```python
from build123d import *

# Parameters (mm, degrees)
F0_R     = 9.5631
F1_DEPTH = 2.5
F2_R     = 8.9162314004
F2_R_2   = 7.9162314004
F3_DEPTH = 0.5
F4_R     = 4
F5_DEPTH = 3.5
F6_R     = 1.2071067812
F7_R     = 1.975
F8_DEPTH = 2.75
F9_R     = 0.4828427125
F10_R    = 0.4587005769


with BuildPart() as f1:
    # F0 (on Top) → F1 (new body)
    with BuildSketch(Plane.XY):
        Circle(F0_R)
    extrude(amount=F1_DEPTH)

    # F2 (on face) → F3 (cut)
    with BuildSketch(Plane.XY.offset(2.5)):
        Circle(F2_R)
        Circle(F2_R_2, mode=Mode.SUBTRACT)
        Polygon((1.8036346717, 5.9258921407), (-2.7067440096, 5.9258921407), (-2.7067440096, 4.4258921407), (-1.8036346717, 4.4258921407), (-1.8036346717, 3.1822535675), (-5.7792644948, 3.1822535675), (-5.7792644948, -4.3527372181), (-4.1694175287, -4.3527372181), (-4.1694175287, -2.3218090646), (-3.4134816378, -2.3218090646), (-3.4134816378, 0), (-1.8036346717, 0), (-2.0609125495, -6.6612055525), (0, -6.6612055525), (2.0609125495, -6.6612055525), (1.8036346717, 0), (3.4134816378, 0), (3.4134816378, -2.3218090646), (4.1694175287, -2.3218090646), (4.1694175287, -4.3527372181), (5.7792644948, -4.3527372181), (5.7792644948, 3.1822535675), (1.8036346717, 3.1822535675), align=None)
    extrude(amount=-F3_DEPTH, mode=Mode.SUBTRACT)

    # F4 (on face) → F5 (join)
    with BuildSketch(Plane(origin=(0, 0, 0), x_dir=(1, 0, 0), z_dir=(0, 0, -1))):
        Circle(F4_R)
    extrude(amount=F5_DEPTH)

    # F6
    f6_edges = [f1.edges().sort_by_distance(p)[0] for p in [
        (-9.5631, 0, 0),
    ]]
    fillet(f6_edges, radius=F6_R)

    # F7 (on face) → F8 (join)
    with BuildSketch(Plane(origin=(0, 0, -3.5), x_dir=(1, 0, 0), z_dir=(0, 0, -1))):
        Circle(F7_R)
    extrude(amount=F8_DEPTH)

    # F9
    f9_edges = [f1.edges().sort_by_distance(p)[0] for p in [
        (-1.975, 0, -6.25),
    ]]
    fillet(f9_edges, radius=F9_R)

    # F10
    f10_edges = [f1.edges().sort_by_distance(p)[0] for p in [
        (-4, 0, -3.5),
    ]]
    fillet(f10_edges, radius=F10_R)


solid = f1.part
```
Check sheet for the modelled part. Datum: model origin and axes. Units: mm. A direction names the side the tool comes from. Round coordinates to 2 decimals unless told otherwise and drop trailing zeros. Order: outer loops, then holes, each group sorted by start corner. A loop starts at its lowest first (then second) coordinate and runs counter-clockwise, first axis right, second up.
1) Tool access check on faces 4 (the cylindrical face through (9.121, 2.872, 1.845)), 5 (the flat face through (4, 2, 0)), 6 (the flat face through (-1.4, 8, 2)). Record the directions out of +Z, -Z, +X, -X, +Y, -Y that give a thin tool (end or side, any length) a straight path to the whole face; none if there is none.
2) Section check A-A (z = 2.25). Record the boundary of the cut face in (x, y), and give its area (3 significant figures).
3) Section check D-D (z = -0.5). Record the boundary of the cut face in (x, y), and give its area (3 significant figures).
4) Mould release check, pull along X, two halves, no side actions. Record for faces 1 (the cylindrical face through (-1.933, -8.704, 2.254)), 2 (the cylindrical face through (-1.57, 1.2, -4.62)), 3 (the flat face through (3, -2, 2.5)): +X half, -X half, draft (parallel to the pull), parting line (faces both ways), or undercut.
5) Go/stop test with flat-tipped pins: pin 1 Ø3 at (x, z) = (2.5, -1) entering from +Y; pin 2 Ø2 at (x, z) = (6.5, -0.5) entering from +Y; pin 3 Ø0.6 at (x, z) = (-5.5, 2.5) entering from +Y. Record where each tip stops, or that it passes through.
6) Section check C-C (z = -4.5). Record the boundary of the cut face in (x, y) (3 decimals), and give its area (3 significant figures).
7) Scan lines: line 1 (Y direction, x = 0, z = 2.3); line 2 (Z direction, x = -2, y = -7.5); line 3 (Z direction, x = -1.25, y = -2.5). Record each from-to range of solid material in increasing order.
Result:
1. face 4: +Z, -Z
1. face 5: -Z
1. face 6: +Z
2. outline: circle Ø19.13 at (0, 0); circle Ø15.83 at (0, 0); hole circle Ø17.83 at (0, 0); hole (-5.78, -4.35) - (-4.17, -4.35) - (-4.17, -2.32) - (-3.41, -2.32) - (-3.41, 0) - (-1.8, 0) - (-2.06, -6.66) - (2.06, -6.66) - (1.8, 0) - (3.41, 0) - (3.41, -2.32) - (4.17, -2.32) - (4.17, -4.35) - (5.78, -4.35) - (5.78, 3.18) - (1.8, 3.18) - (1.8, 5.93) - (-2.71, 5.93) - (-2.71, 4.43) - (-1.8, 4.43) - (-1.8, 3.18) - (-5.78, 3.18) - close
2. area: 143 mm2
3. outline: circle Ø8 at (0, 0)
3. area: 50.3 mm2
4. face 1: undercut
4. face 2: parting line
4. face 3: draft
5. pin 1: stops at y = 9.05
5. pin 2: stops at y = 7.01
5. pin 3: stops at y = 8.03
6. outline: circle Ø3.95 at (0, 0)
6. area: 12.3 mm2
7. line 1: y = -9.56 to -8.92, -7.92 to -6.66, 5.93 to 7.92, 8.92 to 9.56
7. line 2: z = 0 to 2.5
7. line 3: z = -3.5 to 2
